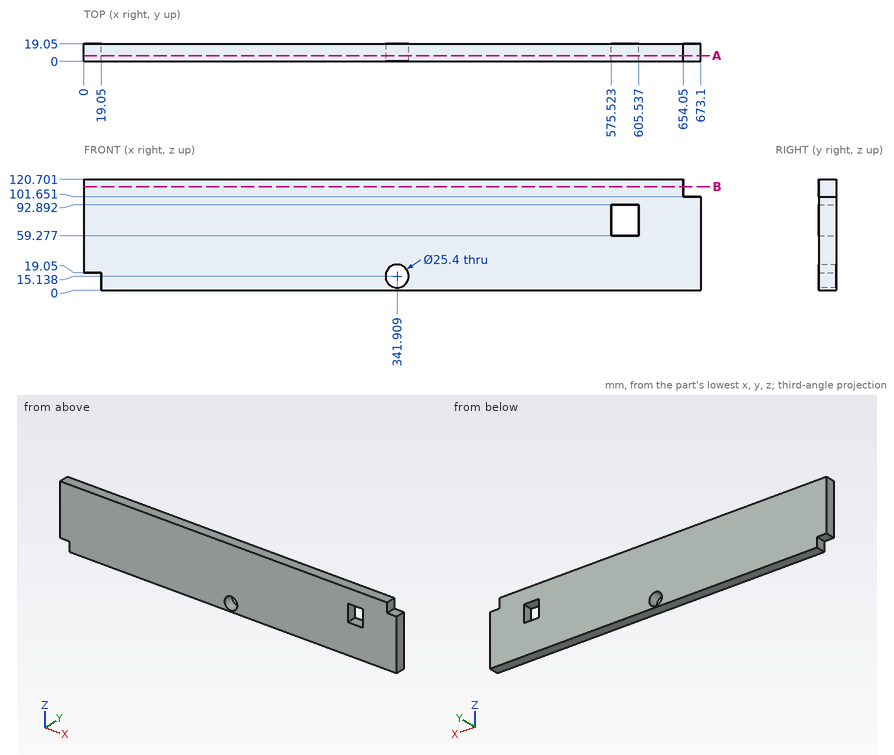
Geometry check sheet. Reference: drawing and pictorial views, mm from the part's lowest x, y, z. Round coordinates to 2 decimals unless told otherwise and drop trailing zeros. Loops run counter-clockwise (first coordinate to the right, second up) from the corner with the lowest first, then second, coordinate; pieces in that order, holes last. Notation, with made-up numbers: (6.5, 9) - (27.5, 9) arc R32 ccw to (27.5, 42) - close; hole circle Ø10 at (23.25, 38.5). An arc over 180 degrees is marked (long way). Use a Markdown table: item, result.
Q1. Material ranges on line 1 (X direction, y = 9, z = 77.5); line 2 (X direction, y = 8, z = 108.5); line 3 (Z direction, x = 581, y = 17.5), recorded low to high.
Solutions:
| item | result |
|---|---|
| line 1 | x = 0 to 575.52, 605.54 to 673.1 |
| line 2 | x = 0 to 654.05 |
| line 3 | z = 0 to 59.28, 92.89 to 120.7 |
Q2. Cross-section at A-A on y = 6.25. Record the cut outline in (x, z).
Solutions:
| item | result |
|---|---|
| outline | (0, 19.05) - (19.05, 19.05) - (19.05, 0) - (673.1, 0) - (673.1, 101.65) - (654.05, 101.65) - (654.05, 120.7) - (0, 120.7) - close; hole circle Ø25.4 at (341.91, 15.14); hole (575.52, 59.28) - (605.54, 59.28) - (605.54, 92.89) - (575.52, 92.89) - close |
Q3. Go/stop test with flat-tipped pins: P1, Ø20.5, axis at x = 341.91, z = 15.14, coming from the +Y side; P2, Ø9.5, axis at y = 6.5, z = 112.5, coming from the +X side. Record where each tip stops, or that it passes through.
Solutions:
| item | result |
|---|---|
| P1 | passes through |
| P2 | stops at x = 654.05 |
Q4. Cross-section at B-B on z = 113. Record the cut outline in (x, y), plus the area to 3 significant figures.
Solutions:
| item | result |
|---|---|
| outline | (0, 0) - (654.05, 0) - (654.05, 19.05) - (0, 19.05) - close |
| area | 12,500 mm2 |
